Geometry: final body of the model. Coordinates: model frame, mm. Face numbers are marked on the shaded views. A direction names the side the tool comes from. Round coordinates to 2 decimals unless told otherwise and drop trailing zeros. Write each loop counter-clockwise with the first axis right and the second up, starting at its lowest first coordinate (ties: lowest second). Pieces come first, ordered by that corner, then holes. Notation, with made-up numbers: (27, -26) -> (62, -26) arc R24 ccw to (62, 12) -> close; hole circle Ø10 at (39, 47.25). An arc over 180 degrees is marked (long way). Use one line per item in the form item = value. Start each with the question number.
1. Reachability of the marked faces 1 and 2 from +Z, -Z, +X, -X, +Y, -Y: full face, straight path, thin tool, end or side. Return the list, or none.
2. Cut plane D-D, the plane x = -85.5. Return the cut outline in (y, z), plus the area to 3 significant figures.
3. Cut plane A-A, the plane z = 20. Return the cut outline in (x, y).
4. Cut plane B-B, the plane z = 123. Return the cut outline in (x, y), plus the area to 3 significant figures.
5. Pin query (flat end, axial travel): pin 1 Ø5 at (x, z) = (-51.08, 144.5) entering from -Y; pin 2 Ø3.5 at (x, z) = (-33.53, 140.5) entering from -Y; pin 3 Ø1.5 at (y, z) = (83.5, 88) entering from -X; pin 4 Ø5 at (y, z) = (90, 52.5) entering from -X. Return the tip coordinate at first contact, or that it passes through.
6. Line query: L1, parallel to X at y = 99, z = 20; L2, parallel to Y at x = -41.5, z = 194; L3, parallel to X at y = 98.45, z = 20. Output: solid intervals per line, ascending.
7. Cut plane C-C, the plane x = -61. Return the cut outline in (y, z).
```python
from build123d import *

# Parameters (mm, degrees)
BASE_FLANGE1_DEPTH = 246
FILLET1_R          = 10
SKETCH7_R          = 3
CUT_EXTRUDE1_DEPTH = 1.5
SKETCH8_R          = 10
SKETCH8_R_2        = 1.6
CUT_EXTRUDE2_DEPTH = 1.5
SKETCH9_R          = 3
CUT_EXTRUDE3_DEPTH = 10


# Sheet-metal steps are written as plain solids
with BuildPart() as part:
    # Sketch1 → Base-Flange1 (new body)
    with BuildSketch(Plane.XY):
        with BuildLine():
            Line((-121.208107966, 98), (-20.950748653, 98))
            ThreePointArc((-20.950748653, 98), (-19.802698356, 97.771638598), (-18.829428309, 97.121320344))
            Line((-18.829428309, 97.121320344), (-3, 81.291892034))
            Line((-3, 81.291892034), (-1.939339828, 82.352552206))
            Line((-1.939339828, 82.352552206), (-17.768768137, 98.181980515))
            ThreePointArc((-17.768768137, 98.181980515), (-19.228673207, 99.157457896), (-20.950748653, 99.5))
            Line((-20.950748653, 99.5), (-121.208107966, 99.5))
            Line((-121.208107966, 99.5), (-121.208107966, 98))
        make_face()
    extrude(amount=BASE_FLANGE1_DEPTH)

    # Fillet1
    fillet1_edges = [part.edges().sort_by_distance(p)[0] for p in [
        (-121.208107966, 98.75, 246),
        (-121.208107966, 98.75, 0),
        (-2.469669914, 81.82222212, 246),
        (-2.469669914, 81.82222212, 0),
    ]]
    fillet(fillet1_edges, radius=FILLET1_R)

    # Sketch7 → Cut-Extrude1 (cut)
    with BuildSketch(Plane(origin=(0, 99.5, 0), x_dir=(1, 0, 0), z_dir=(0, 1, 0))):
        with Locations(Location((-111.208107966, -20, 0), (0, 0, 270))):
            Circle(SKETCH7_R)
        with Locations(Location((-31.208107966, -20, 0), (0, 0, 270))):
            Circle(SKETCH7_R)
        with Locations(Location((-31.208107966, -226, 0), (0, 0, 270))):
            Circle(SKETCH7_R)
        with Locations(Location((-111.208107966, -226, 0), (0, 0, 270))):
            Circle(SKETCH7_R)
    extrude(amount=-CUT_EXTRUDE1_DEPTH, mode=Mode.SUBTRACT)

    # Sketch8 → Cut-Extrude2 (cut)
    with BuildSketch(Plane(origin=(0, 99.5, 0), x_dir=(1, 0, 0), z_dir=(0, 1, 0))):
        with Locations(Location((-66.079428309, -123, 0), (0, 0, 270))):
            Circle(SKETCH8_R)
        with Locations(Location((-51.079428309, -101.5, 0), (0, 0, 270))):
            Circle(SKETCH8_R_2)
        with Locations(Location((-81.079428309, -101.5, 0), (0, 0, 270))):
            Circle(SKETCH8_R_2)
        with Locations(Location((-81.079428309, -144.5, 0), (0, 0, 90))):
            Circle(SKETCH8_R_2)
        with Locations(Location((-51.079428309, -144.5, 0), (0, 0, 90))):
            Circle(SKETCH8_R_2)
    extrude(amount=-CUT_EXTRUDE2_DEPTH, mode=Mode.SUBTRACT)

    # Sketch9 → Cut-Extrude3 (cut)
    with BuildSketch(Plane(origin=(0, 99.5, 0), x_dir=(1, 0, 0), z_dir=(0, 1, 0))):
        with Locations(Location((-33.529428309, -105.5, 0), (0, 0, 270))):
            Circle(SKETCH9_R)
        with Locations(Location((-33.529428309, -140.5, 0), (0, 0, 270))):
            Circle(SKETCH9_R)
        with Locations(Location((-67.198983743, -159.939126893, 0), (0, 0, 270))):
            Circle(SKETCH9_R)
        with Locations(Location((-97.509872875, -142.439126893, 0), (0, 0, 270))):
            Circle(SKETCH9_R)
        with Locations(Location((-97.509872875, -103.560873107, 0), (0, 0, 270))):
            Circle(SKETCH9_R)
        with Locations(Location((-67.198983743, -86.060873107, 0), (0, 0, 270))):
            Circle(SKETCH9_R)
    extrude(amount=-CUT_EXTRUDE3_DEPTH, mode=Mode.SUBTRACT)


solid = part.part
```
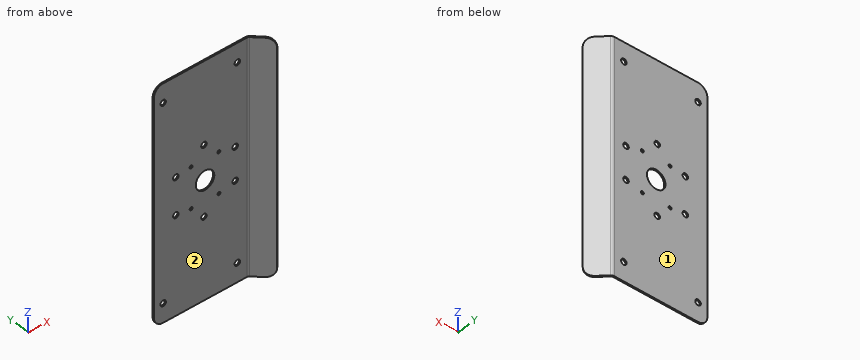
Outcome:
q1.face_1 = +Z, -Z, +X, -X, +Y
q1.face_2 = +Z, -Z, -X, -Y
q2.outline = (98, 0) -> (99.5, 0) -> (99.5, 246) -> (98, 246) -> close
q2.area = 369 mm^2
q3.outline = (-121.21, 98) -> (-114.21, 98) -> (-114.21, 99.5) -> (-121.21, 99.5) -> close; (-108.21, 98) -> (-34.21, 98) -> (-34.21, 99.5) -> (-108.21, 99.5) -> close; (-28.21, 98) -> (-20.95, 98) arc R3 cw to (-18.83, 97.12) -> (-3, 81.29) -> (-1.94, 82.35) -> (-17.77, 98.18) arc R4.5 ccw to (-20.95, 99.5) -> (-28.21, 99.5) -> close
q4.outline = (-121.21, 98) -> (-76.08, 98) -> (-76.08, 99.5) -> (-121.21, 99.5) -> close; (-56.08, 98) -> (-20.95, 98) arc R3 cw to (-18.83, 97.12) -> (-3, 81.29) -> (-1.94, 82.35) -> (-17.77, 98.18) arc R4.5 ccw to (-20.95, 99.5) -> (-56.08, 99.5) -> close
q4.area = 158 mm^2
q5.pin_1 = 98
q5.pin_2 = through
q5.pin_3 = -5.96
q5.pin_4 = -14.21
q6.L1 = -121.21 to -114.21, -108.21 to -34.21, -28.21 to -18.89
q6.L2 = 98 to 99.5
q6.L3 = -121.21 to -114.21, -108.21 to -34.21, -28.21 to -18.06
q7.outline = (98, 0) -> (99.5, 0) -> (99.5, 114.39) -> (98, 114.39) -> close; (98, 131.61) -> (99.5, 131.61) -> (99.5, 246) -> (98, 246) -> close
